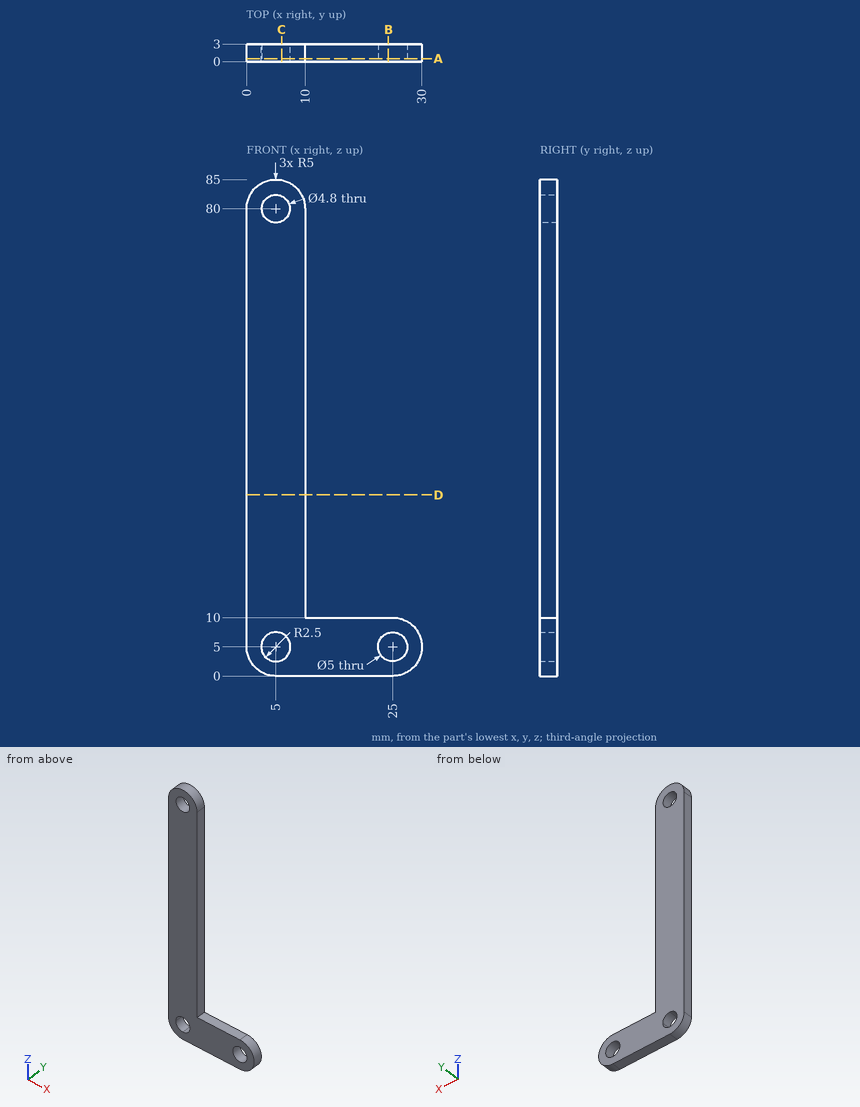
Design review of the part shown in the three views and the two pictorial views. Dimensions are in mm from the part's minimum x, y and z. Round coordinates to 2 decimals unless told otherwise and drop trailing zeros. Write each loop counter-clockwise with the first axis right and the second up, starting at its lowest first coordinate (ties: lowest second). Pieces come first, ordered by that corner, then holes.
Item 1: We need section A-A on y = 0.5. Write out the cut boundary in (x, z).
Item 2: We need section D-D on z = 31. Write out the cut boundary in (x, y), and give its area (3 significant figures).
Item 3: Clearance check with flat-ended pins moving along their axes: pin 1 Ø1 at (x, y) = (18.5, 1.5) entering from +Z; pin 2 Ø1.5 at (y, z) = (1.5, 44.5) entering from +X. State where each tip first meets the part, or that it passes through.
Item 4: We need section C-C on x = 6. Write out the cut boundary in (y, z).
Item 5: For probe 1 along X at (y, z) = (2.3, 5); probe 2 along X at (y, z) = (1.3, 80); probe 3 along X at (y, z) = (2.7, 4), list the stretches that pass through material, from the lowest coordinate up.
Item 6: We need section B-B on x = 24.25. Write out the cut boundary in (y, z).
Returned:
1. outline: (0, 5) arc R5 ccw to (5, 0) - (25, 0) arc R5 ccw to (25, 10) - (10, 10) - (10, 80) arc R5 ccw to (0, 80) - close; hole circle Ø5 at (5, 5); hole circle Ø4.8 at (5, 80); hole circle Ø5 at (25, 5)
2. outline: (0, 0) - (10, 0) - (10, 3) - (0, 3) - close
2. area: 30.0 mm2
3. pin 1: stops at z = 10
3. pin 2: stops at x = 10
4. outline: (0, 0) - (3, 0) - (3, 2.71) - (0, 2.71) - close; (0, 7.29) - (3, 7.29) - (3, 77.82) - (0, 77.82) - close; (0, 82.18) - (3, 82.18) - (3, 84.9) - (0, 84.9) - close
5. probe 1: x = 0 to 2.5, 7.5 to 22.5, 27.5 to 30
5. probe 2: x = 0 to 2.6, 7.4 to 10
5. probe 3: x = 0.1 to 2.71, 7.29 to 22.71, 27.29 to 29.9
6. outline: (0, 0) - (3, 0) - (3, 2.62) - (0, 2.62) - close; (0, 7.38) - (3, 7.38) - (3, 10) - (0, 10) - close
